Model file for the job. Use its own axes, mm. Face numbers are marked on the shaded views. A direction names the side the tool comes from. Round coordinates to 2 decimals unless told otherwise and drop trailing zeros. Order: outer loops, then holes, each group sorted by start corner. A loop starts at its lowest first (then second) coordinate and runs counter-clockwise, first axis right, second up. Notation, with made-up numbers: M 85,35 L 104,35 A22 cw 104,68 Z; hole C -31.75,-4.5 d1. An arc over 180 degrees is marked long. Return JSON: item names as keys, results as strings. Group by question number.
Item 1: Slice it at C-C on y = -59. Write the cut outline in (x, z).
Item 2: Slice it at A-A on x = 0. Give the number of separate pieces and of enclosed holes in the cut face, then the cut area to 3 significant figures.
Item 3: Slice it at B-B on y = 0. Write the cut outline in (x, z) (1 decimal).
Item 4: Pull direction X, two halves, no side cores. Call the marked faces 3, 4 and 5: pulls with the +X half, pulls with the -X half, needs draft (parallel to the pull), parting line crosses it, or undercut.
Item 5: Slice it at D-D on y = -38. Write the cut outline in (x, z).
Item 6: Which spindle directions (+Z, -Z, +X, -X, +Y, -Y) get a long thin tool onto all of the face, cutting with end or side? Do the marked faces 1 and 2. Say none if no direction does.
Item 7: Probe line 1 along Y through (x, z) = (-9, 7); line 2 along Y through (x, z) = (0, 26) (1 decimal); line 3 along Y through (x, z) = (-5, 17.5). List the from-to ranges inside material, lowest first.
Item 8: Pin check, flat tips, straight feed: pin 1 Ø2 at (x, z) = (-21.5, 31) entering from -Y; pin 2 Ø3.5 at (y, z) = (-15, 14) entering from -X; pin 3 Ø4 at (y, z) = (-19.5, 21) entering from -X. Stop position of each tip, or through.
from build123d import *

# Parameters (mm, degrees)
F0_R     = 9.975886
F2_DEPTH = 19.05
F1_R     = 28.575
F3_DEPTH = 45.212
F4_R     = 2.54


with BuildPart() as f2:
    # F0 (on Top) → F2 (new body)
    with BuildSketch(Plane.XY):
        with BuildLine():
            Line((18.923924, -83.46952), (28.575, 0))
            ThreePointArc((28.575, 0), (0, 28.575), (-28.575, 0))
            Line((-28.575, 0), (-18.923924, -83.46952))
            ThreePointArc((-18.923924, -83.46952), (0, -100.331461), (18.923924, -83.46952))
        make_face()
        with Locations((0, -81.281461)):
            Circle(F0_R, mode=Mode.SUBTRACT)
        with BuildLine():
            ThreePointArc((-5.112984, -13.341291), (0.304913, 14.284246), (4.539016, -13.547324))
            Line((4.539016, -13.547324), (4.539016, -17.816696))
            Line((4.539016, -17.816696), (-5.112984, -17.816696))
            Line((-5.112984, -17.816696), (-5.112984, -13.341291))
        make_face(mode=Mode.SUBTRACT)
    extrude(amount=F2_DEPTH)

    # F1 (on Top) → F3 (join)
    with BuildSketch(Plane.XY):
        Circle(F1_R)
        with BuildLine():
            ThreePointArc((-5.112984, -13.341291), (0.304913, 14.284246), (4.539016, -13.547324))
            Line((4.539016, -13.547324), (4.539016, -17.816696))
            Line((4.539016, -17.816696), (-5.112984, -17.816696))
            Line((-5.112984, -17.816696), (-5.112984, -13.341291))
        make_face(mode=Mode.SUBTRACT)
    extrude(amount=F3_DEPTH)

    # F4
    f4_edges = [f2.edges().sort_by_distance(p)[0] for p in [
        (-28.575, 0, 45.212),
    ]]
    fillet(f4_edges, radius=F4_R)


solid = f2.part
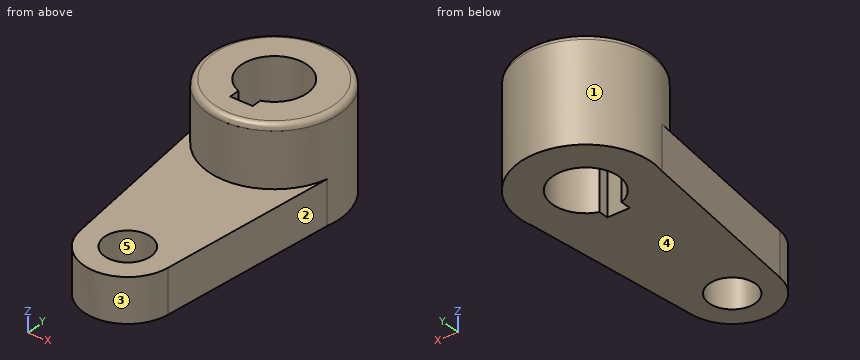
Output values:
{
 "1": {"outline": "M -21.75,0 L 21.75,0 L 21.75,19.05 L -21.75,19.05 Z"},
 "2": {"separate pieces": "3", "enclosed holes": "0", "area": "2,120 mm²"},
 "3": {"outline": "M -28.6,0 L -14.3,0 L -14.3,45.2 L -26,45.2 A2.5 ccw -28.6,42.7 Z; M 14.3,0 L 28.6,0 L 28.6,42.7 A2.5 ccw 26,45.2 L 14.3,45.2 Z"},
 "4": {"face 3": "parting line crosses it", "face 4": "needs draft", "face 5": "undercut"},
 "5": {"outline": "M -24.18,0 L 24.18,0 L 24.18,19.05 L -24.18,19.05 Z"},
 "6": {"face 1": "+Z", "face 2": "+Z, -Z, +X, -Y"},
 "7": {"line 1": "-98.07 to -85.58, -76.98 to -11.1, 11.1 to 27.12", "line 2": "-28.6 to -17.8, 14.3 to 28.6", "line 3": "-99.66 to -89.91, -72.65 to -17.82, 13.38 to 28.13"},
 "8": {"pin 1": "y = -19.91", "pin 2": "x = -27.04", "pin 3": "x = -26.37"}
}
